```python
from build123d import *

# Parameters (mm, degrees)
ESQUISSE1_W             = 80
ESQUISSE1_H             = 80
BOSS_EXTRU_1_DEPTH      = 2
BOSS_EXTRU_2_DEPTH      = 1
ESQUISSE3_R             = 2.05
ESQUISSE3_W             = 78
ESQUISSE3_H             = 3.2
ENL_V_MAT_EXTRU_1_DEPTH = 3
ESQUISSE4_R             = 5
ESQUISSE4_R_2           = 2.05
ENL_V_MAT_EXTRU_2_DEPTH = 4
CHANFREIN1_SIZE         = 1.75
CHANFREIN1_SIZE2        = 2.594481695
CHANFREIN1_PART_2_SIZE  = 1.75
CHANFREIN1_PART_2_SIZE2 = 2.594481695
CHANFREIN1_PART_3_SIZE  = 1.75
CHANFREIN1_PART_3_SIZE2 = 2.594481695
CHANFREIN1_PART_4_SIZE  = 1.75
CHANFREIN1_PART_4_SIZE2 = 2.594481695
ENL_V_MAT_EXTRU_3_DEPTH = 1
ESQUISSE8_R             = 1.25
ENL_V_MAT_EXTRU_4_DEPTH = 3


with BuildPart() as part:
    # Esquisse1 → Boss.-Extru.1 (new body)
    with BuildSketch(Plane.XY):
        with Locations((40, 40)):
            Rectangle(ESQUISSE1_W, ESQUISSE1_H)
    extrude(amount=BOSS_EXTRU_1_DEPTH)

    # Esquisse2 → Boss.-Extru.2 (add)
    with BuildSketch(Plane.XY.offset(2)):
        Polygon((10.1, 6.1), (10.1, 13.1), (3.1, 13.1), (3.1, 69.9), (10.1, 69.9), (10.1, 76.9), (69.9, 76.9), (69.9, 69.9), (76.9, 69.9), (76.9, 13.1), (69.9, 13.1), (69.9, 6.1), align=None)
    extrude(amount=BOSS_EXTRU_2_DEPTH)

    # Esquisse3 → Enlèv. mat.-Extru.1 (cut, through all)
    with BuildSketch(Plane.XY.offset(2)):
        with Locations((5, 75)):
            Circle(ESQUISSE3_R)
        with Locations((75, 75)):
            Circle(ESQUISSE3_R)
        with Locations((75, 8)):
            Circle(ESQUISSE3_R)
        with Locations((5, 8)):
            Circle(ESQUISSE3_R)
        with Locations((40, 1.6)):
            Rectangle(ESQUISSE3_W, ESQUISSE3_H)
    extrude(amount=-ENL_V_MAT_EXTRU_1_DEPTH, mode=Mode.SUBTRACT)

    # Esquisse4 → Enlèv. mat.-Extru.2 (cut, through all)
    with BuildSketch(Plane.XY.offset(3)):
        with Locations((40, 40)):
            Circle(ESQUISSE4_R)
        with Locations((30, 50)):
            Circle(ESQUISSE4_R_2)
        with Locations((30, 30)):
            Circle(ESQUISSE4_R_2)
        with Locations((50, 30)):
            Circle(ESQUISSE4_R_2)
        with Locations((50, 50)):
            Circle(ESQUISSE4_R_2)
    extrude(amount=-ENL_V_MAT_EXTRU_2_DEPTH, mode=Mode.SUBTRACT)

    # Chanfrein1
    chanfrein1_edges = [part.edges().sort_by_distance(p)[0] for p in [
        (2.95, 75, 0),
    ]]
    chanfrein1_side = [part.faces().sort_by_distance(p)[0] for p in [
        (2.95, 75, 1),
    ]]
    chamfer(chanfrein1_edges, length=CHANFREIN1_SIZE, length2=CHANFREIN1_SIZE2, reference=chanfrein1_side[0])

    # Chanfrein1 part 2
    chanfrein1_part_2_edges = [part.edges().sort_by_distance(p)[0] for p in [
        (72.95, 75, 0),
    ]]
    chanfrein1_part_2_side = [part.faces().sort_by_distance(p)[0] for p in [
        (72.95, 75, 1),
    ]]
    chamfer(chanfrein1_part_2_edges, length=CHANFREIN1_PART_2_SIZE, length2=CHANFREIN1_PART_2_SIZE2, reference=chanfrein1_part_2_side[0])

    # Chanfrein1 part 3
    chanfrein1_part_3_edges = [part.edges().sort_by_distance(p)[0] for p in [
        (72.95, 8, 0),
    ]]
    chanfrein1_part_3_side = [part.faces().sort_by_distance(p)[0] for p in [
        (72.95, 8, 1),
    ]]
    chamfer(chanfrein1_part_3_edges, length=CHANFREIN1_PART_3_SIZE, length2=CHANFREIN1_PART_3_SIZE2, reference=chanfrein1_part_3_side[0])

    # Chanfrein1 part 4
    chanfrein1_part_4_edges = [part.edges().sort_by_distance(p)[0] for p in [
        (2.95, 8, 0),
    ]]
    chanfrein1_part_4_side = [part.faces().sort_by_distance(p)[0] for p in [
        (2.95, 8, 1),
    ]]
    chamfer(chanfrein1_part_4_edges, length=CHANFREIN1_PART_4_SIZE, length2=CHANFREIN1_PART_4_SIZE2, reference=chanfrein1_part_4_side[0])

    # Esquisse6 → Enlèv. mat.-Extru.3 (cut)
    with BuildSketch(Plane(origin=(0, 0, 0), x_dir=(-1, 0, 0), z_dir=(0, 0, -1))):
        Polygon((-70.615937957, 56.473802333), (-56.473802333, 70.615937957), (-60.857864376, 75), (-75, 60.857864376), align=None)
    extrude(amount=-ENL_V_MAT_EXTRU_3_DEPTH, mode=Mode.SUBTRACT)

    # Esquisse8 → Enlèv. mat.-Extru.4 (cut, through all)
    with BuildSketch(Plane(origin=(0, 0, 1), x_dir=(-1, 0, 0), z_dir=(0, 0, -1))):
        with Locations((-60.150757595, 71.464466094)):
            Circle(ESQUISSE8_R)
        with Locations((-71.464466094, 60.150757595)):
            Circle(ESQUISSE8_R)
        Polygon((-67.787510832, 59.302229458), (-72.171572875, 63.686291501), (-63.686291501, 72.171572875), (-59.302229458, 67.787510832), align=None)
    extrude(amount=-ENL_V_MAT_EXTRU_4_DEPTH, mode=Mode.SUBTRACT)


solid = part.part
```
Geometry: final body of the model. Coordinates: model frame, mm. A direction names the side the tool comes from. Coordinates: 2 decimals unless noted, no trailing zeros. Order: outer loops, then holes, each group sorted by start corner. A loop starts at its lowest first (then second) coordinate and runs counter-clockwise, first axis right, second up. Notation, with made-up numbers: M 55.5,58 L 62.5,58 A24 cw 62.5,69 Z; hole C 67.25,70.5 d9. An arc over 180 degrees is marked long. Answer in a Markdown table with one row per item. Add a question column.
Q1. Section query A-A on y = 8. Return the cut outline in (x, z), and give its area (3 significant figures).
Q2. Section query C-C on x = 50. Return the cut outline in (y, z), and give its area (3 significant figures).
Q3. Mould query, pull axis Z, two halves, no side actions, for faces 5 (the cylindrical face through (29.733, 32.033, 1.521)), 6 (the flat face through (39, 32, 0)). Classes: released by +Z, released by -Z, zero draft, split by the parting line, or undercut.
Q4. Reachability of faces 1 (the flat face through (79, 2, 1)), 2 (the flat face through (58.5, 71.4, 1)), 3 (the flat face through (80, 39, 1)), 4 (the flat face through (69.949, 61.464, 1.986)) from +Z, -Z, +X, -X, +Y, -Y: full face, straight path, thin tool, end or side. Return the list, or none.
Q5. Section query B-B on x = 5. Return the cut outline in (y, z).
Q6. Contact query for flat-ended pins moving along their axis: P1, Ø0.8, axis at x = 72, z = 2.5, coming from the +Y side; P2, Ø4.5, axis at x = 75, y = 8, coming from the +Z side; P3, Ø0.8, axis at y = 44, z = 2.5, coming from the +X side. Output: stop coordinate, or through.
Q7. Line query: L1, parallel to Y at x = 50, z = 2.1; L2, parallel to Y at x = 50, z = 1.1; L3, parallel to Y at x = 40, z = 1.2. Output: solid intervals per line, ascending.
Q8. Section query D-D on y = 30. Return the cut outline in (x, z), and give its area (3 significant figures).
Completed:
| question | item | result |
|---|---|---|
| 1 | outline | M 0,0 L 0.36,0 L 2.95,1.75 L 2.95,2 L 0,2 Z; M 7.05,1.75 L 9.64,0 L 70.36,0 L 72.95,1.75 L 72.95,2 L 69.9,2 L 69.9,3 L 10.1,3 L 10.1,2 L 7.05,2 Z; M 77.05,1.75 L 79.64,0 L 80,0 L 80,2 L 77.05,2 Z |
| 1 | area | 194 mm2 |
| 2 | outline | M 3.2,0 L 27.95,0 L 27.95,3 L 6.1,3 L 6.1,2 L 3.2,2 Z; M 32.05,0 L 47.95,0 L 47.95,3 L 32.05,3 Z; M 52.05,0 L 80,0 L 80,2 L 76.9,2 L 76.9,3 L 52.05,3 Z |
| 2 | area | 200 mm2 |
| 3 | face 5 | zero draft |
| 3 | face 6 | released by -Z |
| 4 | face 1 | +Z, -Z, -Y |
| 4 | face 2 | -Z |
| 4 | face 3 | +Z, -Z, +X, +Y, -Y |
| 4 | face 4 | +Z, -Z |
| 5 | outline | M 3.2,0 L 3.36,0 L 5.95,1.75 L 5.95,2 L 3.2,2 Z; M 10.05,1.75 L 12.64,0 L 70.36,0 L 72.95,1.75 L 72.95,2 L 69.9,2 L 69.9,3 L 13.1,3 L 13.1,2 L 10.05,2 Z; M 77.05,1.75 L 79.64,0 L 80,0 L 80,2 L 77.05,2 Z |
| 6 | P1 | stops at y = 69.9 |
| 6 | P2 | stops at z = 2 |
| 6 | P3 | stops at x = 76.9 |
| 7 | L1 | y = 6.1 to 27.95, 32.05 to 47.95, 52.05 to 76.9 |
| 7 | L2 | y = 3.2 to 27.95, 32.05 to 47.95, 52.05 to 80 |
| 7 | L3 | y = 3.2 to 35, 45 to 80 |
| 8 | outline | M 0,0 L 27.95,0 L 27.95,3 L 3.1,3 L 3.1,2 L 0,2 Z; M 32.05,0 L 47.95,0 L 47.95,3 L 32.05,3 Z; M 52.05,0 L 80,0 L 80,2 L 76.9,2 L 76.9,3 L 52.05,3 Z |
| 8 | area | 209 mm2 |
